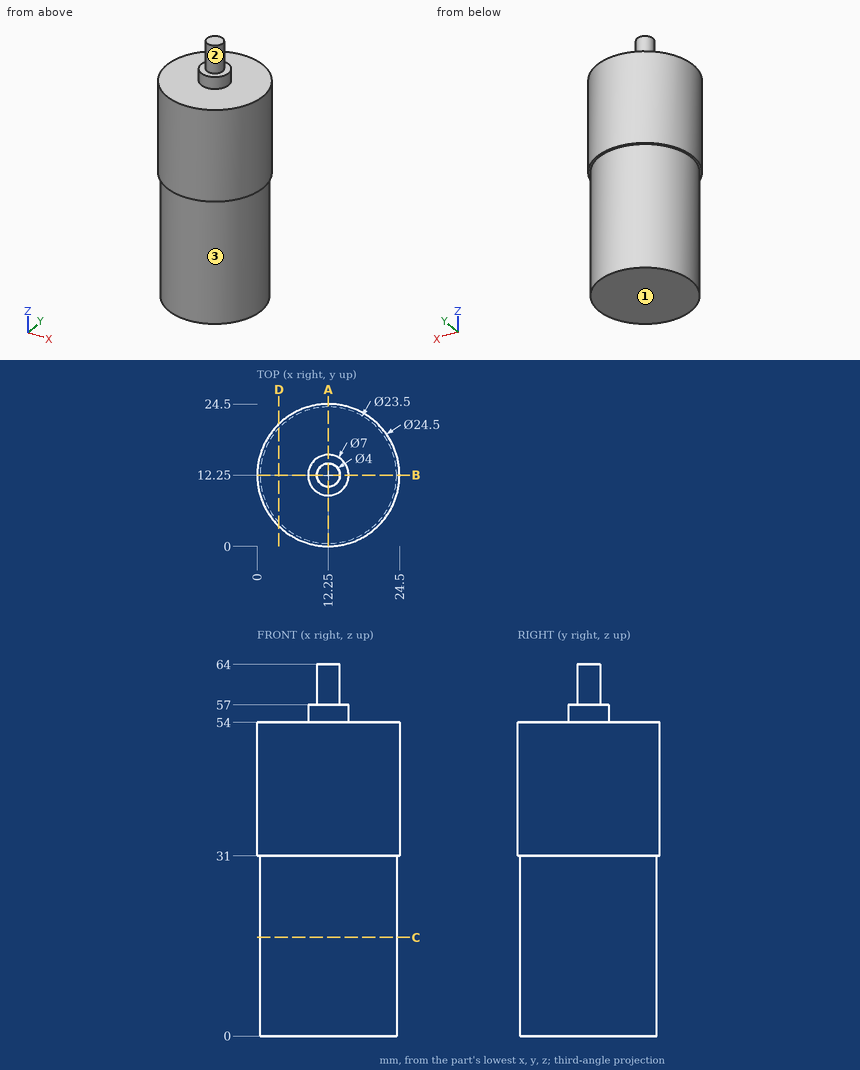
Study the drawing (mm; zero at the part's minimum x, y, z) and answer. A direction names the side the tool comes from. Give positions to 0.01 mm unless a question says otherwise; leave off trailing zeros. Loops run counter-clockwise (first coordinate to the right, second up) from the corner with the lowest first, then second, coordinate; pieces in that order, holes last. Notation, with made-up numbers: (41.25, 47.5) - (98.25, 47.5) arc R34 cw to (98.25, 81.5) - close; hole circle Ø4 at (41.5, -23.75). An arc over 180 degrees is marked (long way). Answer in a Markdown table with one row per item. Add a question column.
Q1. The part is cut by section D-D (x = 3.75). Determine the outline of the cut face in (y, z).
Q2. The part is cut by section A-A (x = 12.25). Determine the outline of the cut face in (y, z), and give its area (3 significant figures).
Q3. A tool of negligible diameter and unlimited length cuts with its end or side. For the marked faces 1, 2 and 3, from which of +Z, -Z, +X, -X, +Y, -Y can it reach the whole face along a straight path? Write none if from no direction.
Q4. Each of these flat-tipped pins is pushed along its axis until it touches: P1, Ø4, axis at y = 3.5, z = 32.5, coming from the -X side; P2, Ø3, axis at x = 3.5, z = 48.5, coming from the -Y side; P3, Ø6, axis at y = 16.5, z = 9.5, coming from the -X side. Where does it stop, or does it pass through?
Q5. Consider line 1 along X through (y, z) = (11.75, 49); line 2 along Z through (x, y) = (5.5, 12.5); line 3 along Z through (x, y) = (1.75, 6.75). Determine where each line is inside the solid, lowest interval first.
Q6. The part is cut by section C-C (z = 17). Determine the outline of the cut face in (x, y).
Solution:
| question | item | result |
|---|---|---|
| 1 | outline | (3.43, 31) - (4.14, 31) - (4.14, 0) - (20.36, 0) - (20.36, 31) - (21.07, 31) - (21.07, 54) - (3.43, 54) - close |
| 2 | outline | (0, 31) - (0.5, 31) - (0.5, 0) - (24, 0) - (24, 31) - (24.5, 31) - (24.5, 54) - (15.75, 54) - (15.75, 57) - (14.25, 57) - (14.25, 64) - (10.25, 64) - (10.25, 57) - (8.75, 57) - (8.75, 54) - (0, 54) - close |
| 2 | area | 1,340 mm² |
| 3 | face 1 | -Z, +X, -X, +Y, -Y |
| 3 | face 2 | +Z |
| 3 | face 3 | -Z |
| 4 | P1 | stops at x = 2.03 |
| 4 | P2 | stops at y = 2.38 |
| 4 | P3 | stops at x = 0.57 |
| 5 | line 1 | x = 0.01 to 24.49 |
| 5 | line 2 | z = 0 to 54 |
| 5 | line 3 | z = 31 to 54 |
| 6 | outline | circle Ø23.5 at (12.25, 12.25) |
